Part model, mm, in its own coordinate system. A direction names the side the tool comes from. Round coordinates to 2 decimals unless told otherwise and drop trailing zeros. Write each loop counter-clockwise with the first axis right and the second up, starting at its lowest first coordinate (ties: lowest second). Pieces come first, ordered by that corner, then holes. Notation, with made-up numbers: M 64.5,67 L 117.5,67 A27 cw 117.5,98 Z; hole C 17,16.25 d9. An arc over 180 degrees is marked long. Use a Markdown table: item, result. Add a question column.
1) Slice it at D-D on y = 40. Write the cut outline in (x, z).
2) Drop flat-ended pins along their axis: P1, Ø2, axis at x = 27, y = 40.5, coming from the +Z side; P2, Ø12, axis at x = 40, z = 14, coming from the -Y side; P3, Ø2.5, axis at y = 21.5, z = -9, coming from the -X side. Give the stop position or say it passes through.
3) Which spindle directions (+Z, -Z, +X, -X, +Y, -Y) get a long thin tool onto all of the face, cutting with end or side? Do faces 1 (the face through (-12.898, 41, 20)), 2 (the face through (-34.905, 41, 15)), 3 (the face through (-7, 38.8, 9)), 4 (the face through (-1, 4, 0)). Say none if no direction does.
4) Slice it at B-B on z = 20.5. Write the cut outline in (x, y).
5) Slice it at C-C on y = 29. Write the cut outline in (x, z).
6) Wall check: probe 1 along X at (y, z) = (40, 28); probe 2 along Y at (x, z) = (19, -6.5); probe 3 along X at (y, z) = (33, -9.5). Give the ranges that are in metal, low to high.
7) Slice it at A-A on z = 1. Write the cut outline in (x, y).
```python
from build123d import *

# Parameters (mm, degrees)
SKETCH2_W           = 100
SKETCH2_H           = 14
BOSS_EXTRUDE1_DEPTH = 4
SKETCH3_W           = 10
SKETCH3_H           = 4
BOSS_EXTRUDE2_DEPTH = 5
SKETCH4_W           = 10
SKETCH4_H           = 5
BOSS_EXTRUDE3_DEPTH = 34.8
SKETCH5_W           = 69.90455619
SKETCH5_H           = 4
BOSS_EXTRUDE4_DEPTH = 54
SKETCH6_W           = 10.347488473
SKETCH6_H           = 44.707321825
CUT_EXTRUDE1_DEPTH  = 14


with BuildPart() as part:
    # Sketch2 → Boss-Extrude1 (new body)
    with BuildSketch(Plane(origin=(0, 0, 0), x_dir=(1, 0, 0), z_dir=(0, 1, 0))):
        Rectangle(SKETCH2_W, SKETCH2_H)
    extrude(amount=BOSS_EXTRUDE1_DEPTH)

    # Sketch3 → Boss-Extrude2 (add)
    with BuildSketch(Plane(origin=(0, 0, -7), x_dir=(-1, 0, 0), z_dir=(0, 0, -1))):
        with Locations((-30, 2)):
            Rectangle(SKETCH3_W, SKETCH3_H)
        with Locations((30, 2)):
            Rectangle(SKETCH3_W, SKETCH3_H)
    extrude(amount=BOSS_EXTRUDE2_DEPTH)

    # Sketch4 → Boss-Extrude3 (add)
    with BuildSketch(Plane(origin=(0, 4, 0), x_dir=(1, 0, 0), z_dir=(0, 1, 0))):
        with Locations((-30, 9.5)):
            Rectangle(SKETCH4_W, SKETCH4_H)
        with Locations((30, 9.5)):
            Rectangle(SKETCH4_W, SKETCH4_H)
    extrude(amount=BOSS_EXTRUDE3_DEPTH)

    # Sketch5 → Boss-Extrude4 (add)
    with BuildSketch(Plane(origin=(0, 0, -12), x_dir=(-1, 0, 0), z_dir=(0, 0, -1))):
        with Locations((-0.047721905, 40.8)):
            Rectangle(SKETCH5_W, SKETCH5_H)
    extrude(amount=-BOSS_EXTRUDE4_DEPTH)

    # Sketch6 → Cut-Extrude1 (cut)
    with BuildSketch(Plane(origin=(0, 42.8, 0), x_dir=(1, 0, 0), z_dir=(0, 1, 0))):
        with Locations((-18.071670011, -19.646339087)):
            Rectangle(SKETCH6_W, SKETCH6_H)
        with Locations((3.92832999, -19.646339087)):
            Rectangle(SKETCH6_W, SKETCH6_H)
        with Locations((25.928329989, -19.646339087)):
            Rectangle(SKETCH6_W, SKETCH6_H)
    extrude(amount=-CUT_EXTRUDE1_DEPTH, mode=Mode.SUBTRACT)


solid = part.part
```
Entries:
| question | item | result |
|---|---|---|
| 1 | outline | M -34.9,-12 L 35,-12 L 35,42 L 31.1,42 L 31.1,-2.71 L 20.75,-2.71 L 20.75,42 L 9.1,42 L 9.1,-2.71 L -1.25,-2.71 L -1.25,42 L -12.9,42 L -12.9,-2.71 L -23.25,-2.71 L -23.25,42 L -34.9,42 Z |
| 2 | P1 | stops at z = -2.71 |
| 2 | P2 | stops at y = 38.8 |
| 2 | P3 | stops at x = -35 |
| 3 | face 1 | +Z, +Y |
| 3 | face 2 | +Z, -Z, -X, +Y |
| 3 | face 3 | +Z |
| 3 | face 4 | +Z, +X, -X |
| 4 | outline | M -34.9,38.8 L -23.25,38.8 L -23.25,42.8 L -34.9,42.8 Z; M -12.9,38.8 L -1.25,38.8 L -1.25,42.8 L -12.9,42.8 Z; M 9.1,38.8 L 20.75,38.8 L 20.75,42.8 L 9.1,42.8 Z; M 31.1,38.8 L 35,38.8 L 35,42.8 L 31.1,42.8 Z |
| 5 | outline | M -35,-12 L -25,-12 L -25,-7 L -35,-7 Z; M 25,-12 L 35,-12 L 35,-7 L 25,-7 Z |
| 6 | probe 1 | x = -34.9 to -23.25, -12.9 to -1.25, 9.1 to 20.75, 31.1 to 35 |
| 6 | probe 2 | y = 0 to 4, 38.8 to 42.8 |
| 6 | probe 3 | x = -35 to -25, 25 to 35 |
| 7 | outline | M -50,0 L 50,0 L 50,4 L -50,4 Z; M -34.9,38.8 L -23.25,38.8 L -23.25,42.8 L -34.9,42.8 Z; M -12.9,38.8 L -1.25,38.8 L -1.25,42.8 L -12.9,42.8 Z; M 9.1,38.8 L 20.75,38.8 L 20.75,42.8 L 9.1,42.8 Z; M 31.1,38.8 L 35,38.8 L 35,42.8 L 31.1,42.8 Z |
